The listing builds one solid part. Answer for the finished solid, in the listing's coordinates (mm). Face numbers are marked on the shaded views. A direction names the side the tool comes from. Round coordinates to 2 decimals unless told otherwise and drop trailing zeros. Order: outer loops, then holes, each group sorted by start corner. A loop starts at its lowest first (then second) coordinate and runs counter-clockwise, first axis right, second up. Notation, with made-up numbers: (69.25, 50.5) -> (108.25, 50.5) arc R17 cw to (108.25, 72.5) -> close; hole circle Ø8 at (-18, 33.25). An arc over 180 degrees is marked (long way). Return JSON: item names as keys, results as strings. Group by question number.
(1) The part is cut by section D-D (x = 20). Determine the outline of the cut face in (y, z).
(2) Each of these flat-tipped pins is pushed along its axis until it touches: pin 1 (17.5 mm diameter, centred on x = 52.5, y = 4, fed in from -Z); pin 2 (1 mm diameter, centred on x = 74.5, y = -9.5, fed in from -Z); pin 3 (5 mm diameter, centred on y = -6.5, z = -9, fed in from -X); pin 4 (2 mm diameter, centred on y = 1.5, z = 1, fed in from +X). Where does it stop, or does it pass through?
(3) The part is cut by section B-B (z = -4). Determine the outline of the cut face in (x, y).
(4) The part is cut by section A-A (z = -29). Determine the outline of the cut face in (x, y), plus the area to 3 significant figures.
(5) Determine the mould class of the marked faces 3, 4 and 5 for opening direction Z: +Z half, -Z half, draft (parallel to the pull), parting line (faces both ways), or undercut.
(6) Which of the six approach directions +Z, -Z, +X, -X, +Y, -Y give full straight-line access (tool end or side, diameter ignored) to the marked faces 1 and 2?
(7) Consider line 1 (Y direction, x = 32.5, z = -28); line 2 (Z direction, x = 75, y = -3); line 3 (X direction, y = -8, z = -28). Determine where each line is inside the solid, lowest interval first. Write a range as [from, to].
(8) The part is cut by section C-C (y = -8). Determine the outline of the cut face in (x, z).
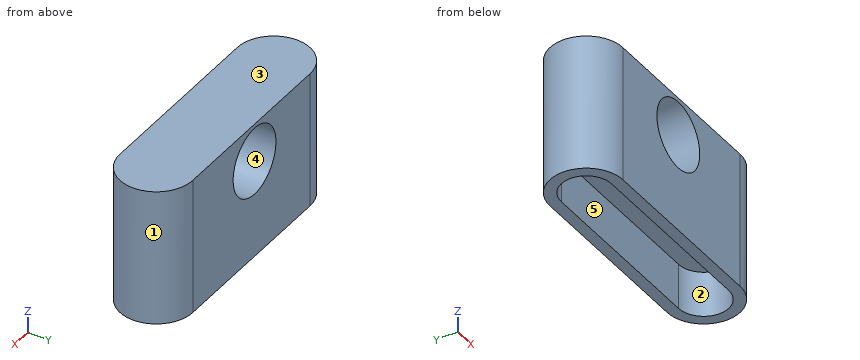
from build123d import *

# Parameters (mm, degrees)
EXTRUDE_1_DEPTH      = 20
EXTRUDE_1_DEPTH_BACK = 20
EXTRUDE_START        = 20
EXTRUDE_1_2_DEPTH    = 20
SKETCH_3_R           = 14.975860866
CUT_EXTRUDE_1_DEPTH  = 111.706390972


with BuildPart() as part:
    # Sketch 1 → Extrude 1 (new, two sides: drawn at the far end of the back side and taken through both)
    with BuildSketch(Plane.XY.offset(-EXTRUDE_1_DEPTH_BACK)):
        with BuildLine():
            Line((0, 16.022995164), (82.104266624, 16.022995164))
            ThreePointArc((82.104266624, 16.022995164), (98.127261788, 0), (82.104266624, -16.022995164))
            Line((82.104266624, -16.022995164), (0, -16.022995164))
            ThreePointArc((0, -16.022995164), (-16.022995164, 0), (0, 16.022995164))
        make_face()
    extrude(amount=EXTRUDE_1_DEPTH + EXTRUDE_1_DEPTH_BACK)

    # Sketch 2 → Extrude 1 2 (add)
    with BuildSketch(Plane(origin=(0, 0, -20), x_dir=(-1, 0, 0), z_dir=(0, 0, -1)).offset(EXTRUDE_START)):
        with BuildLine():
            Line((-82.104266624, -16.022995164), (0, -16.022995164))
            ThreePointArc((0, -16.022995164), (16.022995164, 0), (0, 16.022995164))
            Line((0, 16.022995164), (-82.104266624, 16.022995164))
            ThreePointArc((-82.104266624, 16.022995164), (-98.127261788, 0), (-82.104266624, -16.022995164))
        make_face()
        with BuildLine():
            Line((-82.104266624, -11.022995164), (0, -11.022995164))
            ThreePointArc((0, -11.022995164), (11.022995164, 0), (0, 11.022995164))
            Line((0, 11.022995164), (-82.104266624, 11.022995164))
            ThreePointArc((-82.104266624, 11.022995164), (-93.127261788, 0), (-82.104266624, -11.022995164))
        make_face(mode=Mode.SUBTRACT)
    extrude(amount=-EXTRUDE_1_2_DEPTH)

    # Sketch 3 → Cut-Extrude 1 (cut, through all)
    with BuildSketch(Plane.XZ.offset(16.022995164)):
        with Locations(Location((38.866467132, 3.235422981, 0), (0, 0, 270))):
            Circle(SKETCH_3_R)
    extrude(amount=-CUT_EXTRUDE_1_DEPTH, mode=Mode.SUBTRACT)


solid = part.part
Answer below:
{
 "1": {"outline": "(-16.02, -40) -> (-11.02, -40) -> (-11.02, -20) -> (11.02, -20) -> (11.02, -40) -> (16.02, -40) -> (16.02, 20) -> (-16.02, 20) -> close"},
 "2": {"pin 1": "stops at z = -40", "pin 2": "stops at z = -20", "pin 3": "stops at x = -15.52", "pin 4": "stops at x = 98.12"},
 "3": {"outline": "(0, -16.02) -> (25.75, -16.02) -> (25.75, 16.02) -> (0, 16.02) arc R16.02 ccw to start; (51.98, -16.02) -> (82.1, -16.02) arc R16.02 ccw to (82.1, 16.02) -> (51.98, 16.02) -> close"},
 "4": {"outline": "(0, -16.02) -> (82.1, -16.02) arc R16.02 ccw to (82.1, 16.02) -> (0, 16.02) arc R16.02 ccw to start; hole (0, -11.02) -> (82.1, -11.02) arc R11.02 ccw to (82.1, 11.02) -> (0, 11.02) arc R11.02 ccw to start", "area": "1,250 mm²"},
 "5": {"face 3": "+Z half", "face 4": "undercut", "face 5": "draft"},
 "6": {"face 1": "+Z, -Z, +X", "face 2": "-Z"},
 "7": {"line 1": "y = [-16.02, -11.02], [11.02, 16.02]", "line 2": "z = [-20, 20]", "line 3": "x = [-13.88, -7.58], [89.69, 95.99]"},
 "8": {"outline": "(-13.88, -40) -> (-7.58, -40) -> (-7.58, -20) -> (89.69, -20) -> (89.69, -40) -> (95.99, -40) -> (95.99, 20) -> (-13.88, 20) -> close; hole circle Ø29.95 at (38.87, 3.24)"}
}
